```python
from build123d import *

# Parameters (mm, degrees)
F0_R     = 10
F1_DEPTH = 101.6
F4_R     = 38.1
F5_DEPTH = 12.7
F6_R     = 4.25
F7_DEPTH = 15
F8_R     = 38.1
F8_R_2   = 25.4
F9_DEPTH = 25.4


with BuildPart() as f1:
    # F0 (on Top) → F1 (new body)
    with BuildSketch(Plane.XY):
        Circle(F0_R)
    extrude(amount=F1_DEPTH)

    # F2 (on Front) → F3 (revolve)
    with BuildSketch(Plane.XZ):
        with BuildLine():
            Line((0, 101.6), (0, 0))
            Line((0, 0), (7.7706216834, 0))
            add(Edge.make_bspline(
                [(38.1, 101.6), (33.7451557732, 101.056594794), (17.7116021292, 99.0558994609), (11.960024104, 41.7448789118), (7.7706216834, 0)],
                knots=[0, 0, 0, 0, 0.2716081739, 1, 1, 1, 1], degree=3))
            Line((38.1, 101.6), (0, 101.6))
        make_face()
    revolve(axis=Axis((0, 0, 50.8), (0, 0, 1)))

    # F4 (on face) → F5 (join)
    with BuildSketch(Plane.XY.offset(101.6)):
        Circle(F4_R)
    extrude(amount=F5_DEPTH)

    # F6 (on face) → F7 (cut)
    with BuildSketch(Plane(origin=(0, 0, 0), x_dir=(1, 0, 0), z_dir=(0, 0, -1))):
        Circle(F6_R)
    extrude(amount=-F7_DEPTH, mode=Mode.SUBTRACT)

    # F8 (on face) → F9 (cut)
    with BuildSketch(Plane.XY.offset(114.3)):
        Circle(F8_R)
        Circle(F8_R_2, mode=Mode.SUBTRACT)
    extrude(amount=-F9_DEPTH, mode=Mode.SUBTRACT)


solid = f1.part
```
Could you check a few things on this model? Use its own coordinates, in mm. A direction names the side the tool comes from. Coordinates: 2 decimals unless noted, no trailing zeros. Loops run counter-clockwise (first coordinate to the right, second up) from the corner with the lowest first, then second, coordinate; pieces in that order, holes last. Notation, with made-up numbers: M 34.25,-21 L 69.25,-21 A20 cw 69.25,1 Z; hole C -28,88.5 d5. An arc over 180 degrees is marked long. Put each result on its own line as item: value. Start each with the question number.
(1) Suppose I cut it at A-A on z = 11.5. Please give me the cut outline in (x, y), then the cut area to 3 significant figures.
(2) Will these pins go through, and if not, where does the flat tip stop? P1, Ø6, axis at y = -16, z = 62.5, coming from the -X side; P2, Ø10, axis at x = 9, z = 49.5, coming from the +Y side; P3, Ø4, axis at x = 1, y = 1, coming from the -Z side; P4, Ø2, axis at x = -14, z = 31.5, coming from the +Y side.
(3) For faces 4 (the face through (2.285, -3.584, 7.395)), 5 (the face through (0, 0, 114.3)), which set-ups out of +Z, -Z, +X, -X, +Y, -Y let a thin tool reach every point of the face, with its end or its side?
(4) Thinking about a two-plate mould opening in X: for faces 1 (the face through (-2.17, -9.76, 10.73)), 2 (the face through (0, 0, 15)), 3 (the face through (2, -4, 0)), which applies, pulls with the +X half, pulls with the -X half, needs draft (parallel to the pull), parting line crosses it, or undercut?
(5) I need wall thicknesses on line 1 (Y direction, x = 0, z = 10); line 2 (Z direction, x = -1, y = -3.5). Which ranges of each line are inside material? Lowest first, please. Write a range as from..to.
Solutions:
1. outline: C 0,0 d20; hole C 0,0 d8.5
1. area: 257 mm2
2. P1: stops at x = -8.22
2. P2: stops at y = 12.87
2. P3: stops at z = 15
2. P4: passes through
3. face 4: -Z
3. face 5: +Z, +X, -X, +Y, -Y
4. face 1: parting line crosses it
4. face 2: undercut
4. face 3: needs draft
5. line 1: y = -10..-4.25, 4.25..10
5. line 2: z = 15..114.3
